Source: CAD feature listing. Evaluate the final solid. Frame: model axes, mm. Face numbers are marked on the shaded views. A direction names the side the tool comes from. Give positions to 0.01 mm unless a question says otherwise; leave off trailing zeros. Order: outer loops, then holes, each group sorted by start corner. A loop starts at its lowest first (then second) coordinate and runs counter-clockwise, first axis right, second up. Notation, with made-up numbers: M 83,81 L 138,81 A18 ccw 138,116 Z; hole C 45,51.5 d6. An arc over 180 degrees is marked long. Answer in a Markdown table with one row per item. Add a question column.
(1) Section query B-B, the plane z = -19. Return loops of the section in (x, y) (1 decimal).
(2) Pin query (flat end, axial travel): P1, Ø1.3, axis at x = 0.5, z = -1, coming from the +Y side; P2, Ø0.8, axis at x = -0.5, z = -0.5, coming from the -Y side; P3, Ø6, axis at x = -3, z = -17.5, coming from the +Y side. Return the tip coordinate at first contact, or that it passes through.
(3) Set-up query: the marked faces 1, 2 and 3. Return all of +Z, -Z, +X, -X, +Y, -Y with unobstructed straight access to the full face (end or side cutting, diameter ignored); none if empty.
(4) Material intervals for line 1 along Z through (x, y) = (-3, -2.25) (3 decimals); line 2 along Z through (x, y) = (-2, 2.75) (3 decimals); line 3 along Y through (x, z) = (-2.75, -21), sorted ascending.
(5) Mould query, pull axis Z, two halves, no side actions, for the marked faces 4, 5 and 6. Classes: pulls with the +Z half, pulls with the -Z half, needs draft (parallel to the pull), parting line crosses it, or undercut.
from build123d import *

# Parameters (mm, degrees)
F3_DEPTH = 1.5875


with BuildPart() as f1:
    # F0 (on Front) → F1 (revolve)
    with BuildSketch(Plane.XZ):
        Polygon((5.3441451588, 0), (0, 0), (0, -3.2258), (0, -41.275), (2.54, -41.275), (2.54, -34.925), (4.7625, -34.925), (4.7625, -6.35), (2.54, -6.35), (2.54, -3.2258), align=None)
    revolve(axis=Axis((0, 0, -22.2504), (0, 0, -1)))

    # F2 (on face) → F3 (cut)
    with BuildSketch(Plane.XY):
        Polygon((0.9165435523, 1.5875), (-0.9165435523, 1.5875), (-1.8330871047, 0), (-0.9165435523, -1.5875), (0.9165435523, -1.5875), (1.8330871047, 0), align=None)
    extrude(amount=-F3_DEPTH, mode=Mode.SUBTRACT)


solid = f1.part
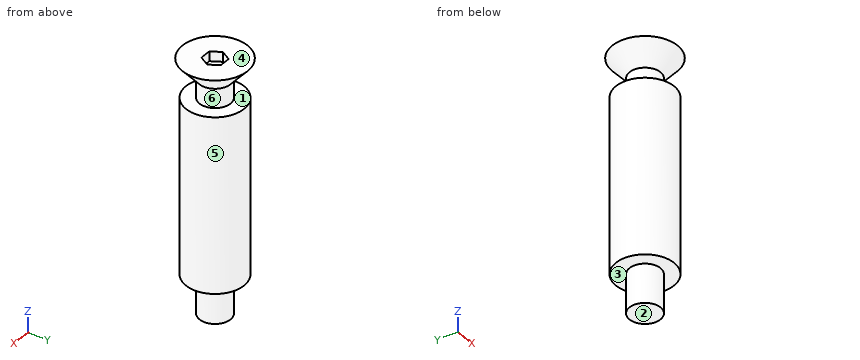
Values follow:
| question | item | result |
|---|---|---|
| 1 | outline | C 0,0 d9.5 |
| 2 | P1 | stops at y = 5.02 |
| 2 | P2 | stops at y = -5.24 |
| 2 | P3 | stops at y = 4.76 |
| 3 | face 1 | none |
| 3 | face 2 | -Z, +X, -X, +Y, -Y |
| 3 | face 3 | -Z |
| 4 | line 1 | z = -34.925 to -6.35, -1.834 to 0 |
| 4 | line 2 | z = -34.925 to -6.35, -2.236 to 0 |
| 4 | line 3 | y = -3.89 to 3.89 |
| 5 | face 4 | pulls with the +Z half |
| 5 | face 5 | needs draft |
| 5 | face 6 | undercut |
